Autodesk Inventor part; units mm, degrees
ref_plane "YZ Plane" through (0, 0, 0) normal (1, 0, 0) x (0, 1, 0)
ref_plane "XZ Plane" through (0, 0, 0) normal (0, 1, 0) x (-1, 0, 0)
ref_plane "XY Plane" through (0, 0, 0) normal (0, 0, 1) x (1, 0, 0)
sketch "Sketch1" plane through (0, 0, 0) normal (0, 1, 0) x (-1, 0, 0)
  line L0 (17.5, 0) -> (-17.5, 0) construction
  line L1 (17.5, 3.5) -> (-17.5, 3.5)
  line L2 (-17.5, -3.5) -> (17.5, -3.5)
  arc A0 (17.5, -3.5) -> (17.5, 3.5) centre (17.5, 0) ccw
  arc A1 (-17.5, 3.5) -> (-17.5, -3.5) centre (-17.5, 0) ccw
  circle A2 centre (-17.5, 0) radius 1.75
  circle A3 centre (17.5, 0) radius 1.75
  circle A4 centre (0, 0) radius 14
  dimension "d0" = 17.5
  dimension "d1" = 7
  dimension "d2" = 3.5
  dimension "d3" = 3.5
  dimension "d4" = 28
extrude "Extrusion1" add sketch "Sketch1" against normal blind 0.8
sketch "Sketch2" plane through (0, 0, 0) normal (0, 1, 0) x (1, 0, 0)
  arc A0 (-13.5554, -3.5) -> (13.5554, -3.5) centre (0, 0) ccw
  line L0 (17.5, 3.5) -> (13.5554, 3.5)
  line L1 (0, 0) -> (0, 8)
  line L2 (0, 0) -> (8, 0) construction
  circle A1 centre (0, 8) radius 4.5
  dimension "d7" = 8
  dimension "d8" = 90
  dimension "d9" = 9
extrude "Extrusion2" add sketch "Sketch2" along normal blind 1.5
sketch "Sketch3" plane through (0, 1.5, -8) normal (0, 1, 0) x (1, 0, 0)
  circle A0 centre (0, 0) radius 4.5
  circle A1 centre (0, 0) radius 2.5
  point P0 (0, -8)
  dimension "d12" = 5
extrude "Extrusion3" [suppressed]
sketch "Sketch4" plane through (0, 4, -8) normal (0, 1, 0) x (1, 0, 0)
  circle A0 centre (0, 0) radius 2.5
  line L0 (2, -1.5) -> (-2, -1.5)
  line L1 (-2, -1.5) -> (-2, 1.5)
  line L2 (-2, 1.5) -> (2, 1.5)
  line L3 (2, 1.5) -> (2, -1.5)
  line L4 (2, -1.5) -> (-2, 1.5) construction
  line L5 (-2, -1.5) -> (2, 1.5) construction
  arc A1 (-2, 1.5) -> (-2, -1.5) centre (0, 0) ccw
  arc A2 (2, 1.5) -> (-2, 1.5) centre (0, 0) ccw
  arc A3 (2, -1.5) -> (2, 1.5) centre (0, 0) ccw
  arc A4 (-2, -1.5) -> (2, -1.5) centre (0, 0) ccw
  point P0 (0, -8)
  dimension "d15" = 3
extrude "Extrusion4" [suppressed]
sketch "Sketch5" plane through (0, -0.8, 0) normal (0, -1, 0) x (1, 0, 0)
  arc A0 (13.5554, 3.5) -> (-13.5554, 3.5) centre (0, 0) ccw
  circle A1 centre (0, 0) radius 14
  dimension "d18" = 28
extrude "Extrusion5" add sketch "Sketch5" along normal blind 19
equation "\"wood_thickness\" = 5.08"
equation "\"m3_diameter\" = 3.15"
equation "\"m5_diameter\" = 5.25"
equation "\"stepper_screw_space\" = 35"
equation "\"stepper_shaft_diameter\" = 5"
equation "\"stepper_body_diameter\" = 28"
equation "\"laser_body_diameter\" = 12"
properties part number "small_stepper" material "Bronze, Cast"
Geometry: final body of the model. Coordinates: model frame, mm. A direction names the side the tool comes from. Round coordinates to 2 decimals unless told otherwise and drop trailing zeros. Order: outer loops, then holes, each group sorted by start corner. A loop starts at its lowest first (then second) coordinate and runs counter-clockwise, first axis right, second up. Notation, with made-up numbers: (54, -6) -> (68, -6) arc R20 cw to (68, 6) -> close; hole circle Ø10 at (-25.5, 35.25). An arc over 180 degrees is marked (long way). Put each result on its own line as item: value. Start each with the question number.
Q1. Section C-C on x = -18. Return the cut outline in (y, z), and give its area (3 significant figures).
Q2. Line query: probe 1 along Z at (x, y) = (-17.5, -0.35); probe 2 along Y at (x, z) = (-13, 2.5); probe 3 along Y at (x, z) = (-14, -1). Output: solid intervals per line, ascending.
Q3. Section B-B on x = 0. Return the cut outline in (y, z), and give its area (3 significant figures).
Q4. Section D-D on z = -4.5. Return the cut outline in (x, y), and give its area (3 significant figures).
Q5. First-contact query: pin 1 (10 mm diameter, centred on x = -8.5, z = 8.5, fed in from +Y); pin 2 (2 mm diameter, centred on x = -17.5, z = 0, fed in from -Y); pin 3 (3.5 mm diameter, centred on x = -16.5, z = 0, fed in from -Y); pin 4 (5 mm diameter, centred on y = -16, z = -5.5, fed in from -X). Flat tips, straight axial feed; report the tip coordinate or a pass-through.
Q6. Section A-A on z = 0. Return the cut outline in (x, y), and give its area (3 significant figures).
Q7. Reachability of faces 1 (the cylindrical face through (-0.98, 0.74, -12.39)), 2 (the flat face through (0, -19.8, 0)) from +Z, -Z, +X, -X, +Y, -Y: full face, straight path, thin tool, end or side. Return the list, or none.
Q8. Pull-direction query (X, two-part tool) for faces 3 (the flat face through (0, 1.5, -8)), 4 (the cylindrical face through (-16.11, -0.39, -1.06)), 5 (the cylindrical face through (0, -10, -14)); classes: +X half, -X half, draft (parallel to the pull), parting line (faces both ways), or undercut.
Ans:
1. outline: (-0.8, -3.46) -> (0, -3.46) -> (0, -1.68) -> (-0.8, -1.68) -> close; (-0.8, 1.68) -> (0, 1.68) -> (0, 3.46) -> (-0.8, 3.46) -> close
1. area: 2.86 mm2
2. probe 1: z = -3.5 to -1.75, 1.75 to 3.5
2. probe 2: y = -19.8 to 0
2. probe 3: y = -0.8 to 0
3. outline: (-19.8, -14) -> (0, -14) -> (0, -12.5) -> (1.5, -12.5) -> (1.5, -3.5) -> (0, -3.5) -> (0, 14) -> (-19.8, 14) -> close
3. area: 568 mm2
4. outline: (-13.26, -19.8) -> (13.26, -19.8) -> (13.26, 0) -> (2.83, 0) -> (2.83, 1.5) -> (-2.83, 1.5) -> (-2.83, 0) -> (-13.26, 0) -> close
4. area: 533 mm2
5. pin 1: stops at y = 0
5. pin 2: passes through
5. pin 3: stops at y = -0.8
5. pin 4: stops at x = -13.67
6. outline: (-21, -0.8) -> (-19.25, -0.8) -> (-19.25, 0) -> (-21, 0) -> close; (-15.75, -0.8) -> (-14, -0.8) -> (-14, -19.8) -> (14, -19.8) -> (14, -0.8) -> (15.75, -0.8) -> (15.75, 0) -> (-15.75, 0) -> close; (19.25, -0.8) -> (21, -0.8) -> (21, 0) -> (19.25, 0) -> close
6. area: 560 mm2
7. face 1: +Y
7. face 2: +Z, -Z, +X, -X, -Y
8. face 3: draft
8. face 4: undercut
8. face 5: parting line
